Geometry: see drawing. Coordinates: mm, zero at the bounding-box minimum. Coordinates: 2 decimals unless noted, no trailing zeros. Write each loop counter-clockwise with the first axis right and the second up, starting at its lowest first coordinate (ties: lowest second). Pieces come first, ordered by that corner, then holes. Notation, with made-up numbers: (7.5, -28) -> (17.5, -28) arc R23 ccw to (17.5, 3) -> close; hole circle Ø9 at (-17.75, 36). An arc over 180 degrees is marked (long way). Answer as a JSON object with one key per item and string values. Group by question number.
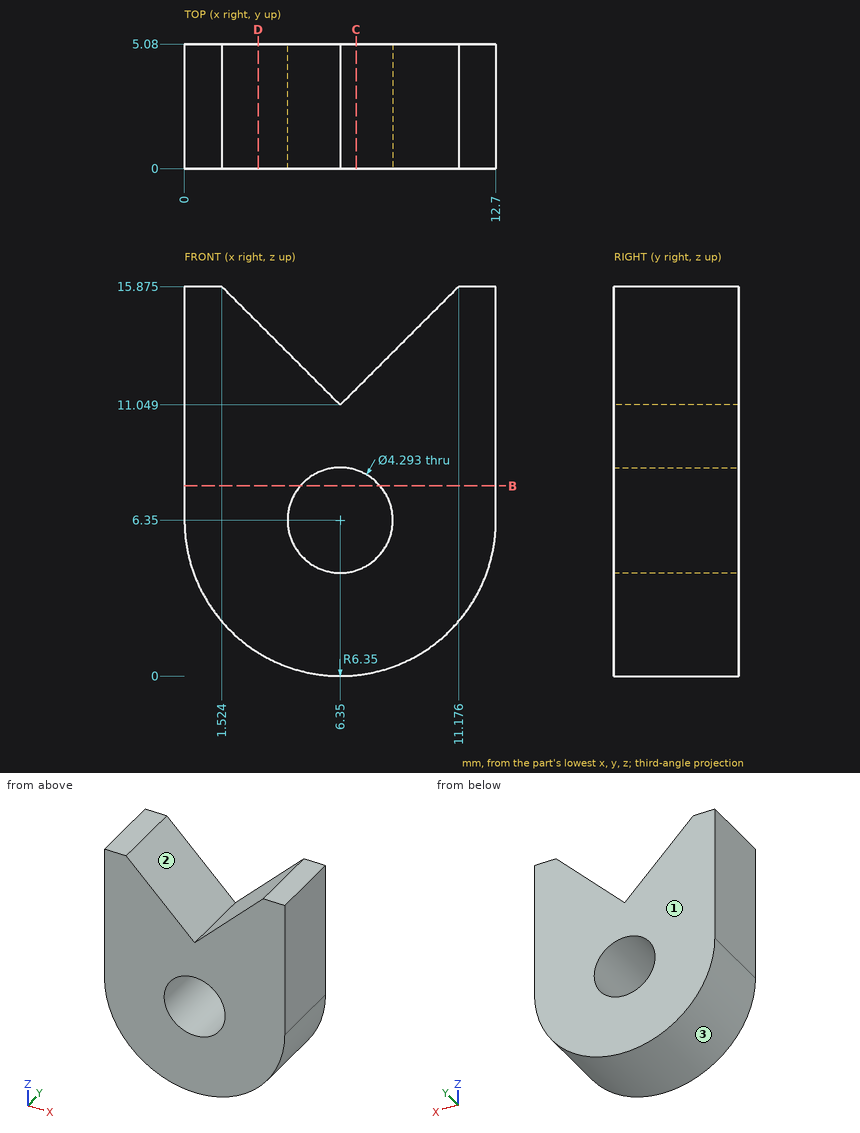
Item 1: Mould query, pull axis X, two halves, no side actions, for the marked faces 1, 2 and 3. Classes: +X half, -X half, draft (parallel to the pull), parting line (faces both ways), or undercut.
Item 2: Section C-C on x = 7. Output: boundary loops of the cut face in (y, z) (1 decimal), then the cut area to 3 significant figures.
Item 3: Ray query, L1, parallel to Z at x = 5.75, y = 1.45; L2, parallel to X at y = 1.8, z = 6; L3, parallel to Z at x = 5, y = 3.6 (1 decimal). Return the intervals inside material, ascending. Write a range as [from, to].
Item 4: Section D-D on x = 3. Output: boundary loops of the cut face in (y, z) (1 decimal).
Item 5: Section B-B on z = 7.75. Output: boundary loops of the cut face in (x, y), then the cut area to 3 significant figures.
Item 6: Contact query for flat-ended pins moving along their axis: pin 1 (2 mm diameter, centred on x = 11, y = 3, fed in from -Z) (1 decimal); pin 2 (3 mm diameter, centred on x = 8, y = 1.5, fed in from -Z). Output: stop coordinate, or through.
Answer sheet:
{
 "1": {"face 1": "draft", "face 2": "undercut", "face 3": "parting line"},
 "2": {"outline": "(0, 0) -> (5.1, 0) -> (5.1, 4.3) -> (0, 4.3) -> close; (0, 8.4) -> (5.1, 8.4) -> (5.1, 11.7) -> (0, 11.7) -> close", "area": "38.5 mm^2"},
 "3": {"L1": "z = [0.03, 4.29], [8.41, 11.65]", "L2": "x = [0.01, 4.23], [8.47, 12.69]", "L3": "z = [0.1, 4.7], [8, 12.4]"},
 "4": {"outline": "(0, 1) -> (5.1, 1) -> (5.1, 14.4) -> (0, 14.4) -> close"},
 "5": {"outline": "(0, 0) -> (4.72, 0) -> (4.72, 5.08) -> (0, 5.08) -> close; (7.98, 0) -> (12.7, 0) -> (12.7, 5.08) -> (7.98, 5.08) -> close", "area": "48.0 mm^2"},
 "6": {"pin 1": "stops at z = 1.2", "pin 2": "stops at z = 0"}
}
